Autodesk Fusion 360 part; units mm, degrees
sketch "Sketch1" plane through (0, 0, 0) normal (0, 0, 1) x (1, 0, 0)
  line L0 (0, 0) -> (100, 0)
  line L1 (100, 0) -> (100, 100)
  line L2 (100, 100) -> (0, 100)
  line L3 (0, 100) -> (0, 0)
  line L4 (0, 0) -> (15, 0)
  line L5 (15, 0) -> (15, 15)
  line L6 (100, 100) -> (85, 100)
  line L7 (85, 100) -> (85, 85)
  line L8 (15, 15) -> (85, 15)
  line L9 (85, 15) -> (85, 85)
  line L10 (85, 85) -> (15, 85)
  line L11 (15, 85) -> (15, 15)
  dimension "d1" = 100
  dimension "d2" = 100
  dimension "d3" = 15
  dimension "d4" = 15
  dimension "d5" = 15
  dimension "d6" = 15
extrude "Extrude1" add sketch "Sketch1" along normal blind 5 contours L0 L2 L3 L4 L5 L7 L10 L11 | L0 L1 L2 L5 L6 L7 L8 L9
chamfer "Chamfer1" distance 5 angle 45 1 edges at (50, 0, 5)
chamfer "Chamfer2" distance 5 angle 45 1 edges at (0, 52.5, 5)
chamfer "Chamfer3" distance 5 angle 45 1 edges at (52.5, 100, 5)
chamfer "Chamfer4" distance 5 angle 45 1 edges at (100, 50, 5)
extrude "Extrude2" cut 1 faces at (5, 61.6667, 0) along direction (0, 0, 1) blind 3
sketch "Sketch2" plane through (0, 0, 5) normal (0, 0, 1) x (-1, 0, 0)
  line L0 (-15, -15) -> (-15, -85)
  line L1 (-15, -85) -> (-85, -85)
  line L2 (-85, -85) -> (-85, -15)
  line L3 (-85, -15) -> (-15, -15)
  line L4 (-95, -5) -> (-95, -95)
  line L5 (-95, -95) -> (-5, -95)
  line L6 (-5, -95) -> (-5, -5)
  line L7 (-5, -5) -> (-95, -5)
  circle A0 centre (-10, -90) radius 2.5
  line L8 (-10, -90) -> (-20, -90)
  circle A1 centre (-20, -90) radius 2.5
  line L9 (-10, -90) -> (-10, -80)
  circle A2 centre (-10, -80) radius 2.5
  circle A3 centre (-90, -90) radius 2.5
  line L10 (-90, -90) -> (-90, -80)
  line L11 (-90, -90) -> (-80, -90)
  circle A4 centre (-90, -80) radius 2.5
  circle A5 centre (-80, -90) radius 2.5
  circle A6 centre (-90, -10) radius 2.5
  line L12 (-90, -10) -> (-90, -20)
  line L13 (-90, -10) -> (-80, -10)
  circle A7 centre (-80, -10) radius 2.5
  circle A8 centre (-90, -20) radius 2.5
  circle A9 centre (-10, -10) radius 2.5
  line L14 (-10, -10) -> (-20, -10)
  line L15 (-10, -10) -> (-10, -20)
  circle A10 centre (-20, -10) radius 2.5
  circle A11 centre (-10, -20) radius 2.5
  dimension "d15" = 5
  dimension "d16" = 10
  dimension "d17" = 5
  dimension "d18" = 10
  dimension "d19" = 5
  dimension "d20" = 5
  dimension "d21" = 10
  dimension "d22" = 10
  dimension "d23" = 5
  dimension "d24" = 5
  dimension "d25" = 5
  dimension "d26" = 10
  dimension "d27" = 10
  dimension "d28" = 5
  dimension "d29" = 5
  dimension "d30" = 5
  dimension "d31" = 10
  dimension "d32" = 10
  dimension "d33" = 5
  dimension "d34" = 5
extrude "Extrude3" cut sketch "Sketch2" against normal blind 5 contours A0 L8 L9 | A1 | A2 | A0 L8 L9 | A3 L10 L11 | A4 | A3 L10 L11 | A5 | A6 L12 L13 | A8 | A6 L12 L13 | A7 | A9 L14 L15 | A11 | A10 | A9 L14 L15
fillet "Fillet1" radius 5 1 edges at (15, 85, 4)
fillet "Fillet2" radius 5 1 edges at (85, 15, 4)
fillet "Fillet3" radius 5 1 edges at (15, 15, 4)
fillet "Fillet4" radius 5 1 edges at (85, 85, 4)
Build history of the part. All positions in model axes, mm. A direction names the side the tool comes from. Coordinates: 2 decimals unless noted, no trailing zeros. Order: outer loops, then holes, each group sorted by start corner. A loop starts at its lowest first (then second) coordinate and runs counter-clockwise, first axis right, second up. Notation, with made-up numbers: M 18.25,-39 L 50.25,-39 A34 cw 50.25,-1 Z; hole C 30,54.25 d3. An arc over 180 degrees is marked long. One line per question, with ' | ' between items. Start each with the question number.
1. Cut at A-A (x = 57). Write the cut outline in (y, z), plus the area to 3 significant figures.
2. Cut at C-C (x = 90). Write the cut outline in (y, z).
3. Mould opens along Y. For faces 1 (the face through (51, 4, 4)), 2 (the face through (49, 96, 4)), 3 (the face through (92.5, 79.9, 4)) say: +Y half, -Y half, draft (parallel to the pull), parting line (faces both ways), or undercut.
4. Tool access for faces 4 (the face through (4, 49, 4)), 5 (the face through (17, 84, 4)): list every direction of +Z, -Z, +X, -X, +Y, -Y with a clear straight run to the whole face (end or side of a thin tool).
5. Wall check: line 1 along X through (y, z) = (10, 4.9); line 2 along X through (y, z) = (20.5, 3.95); line 3 along X through (y, z) = (10, 3.65). Give the ranges that are in metal, low to high. Write a range as [from, to].
6. Flat gauge pins, fed straight in: P1, Ø3, axis at x = 90, y = 10, coming from the +Z side; P2, Ø0.6, axis at y = 40, z = 4, coming from the +X side; P3, Ø0.6, axis at y = 44, z = 3.5, coming from the -X side; P4, Ø0.6, axis at x = 45, z = 4, coming from the -Y side. Where does each tip first touch, or does it go through?
The answers:
1) outline: M 3,3 L 15,3 L 15,5 L 5,5 Z; M 85,3 L 97,3 L 95,5 L 85,5 Z | area: 44.0 mm2
2) outline: M 3,3 L 7.5,3 L 7.5,5 L 5,5 Z; M 12.5,3 L 17.5,3 L 17.5,5 L 12.5,5 Z; M 22.5,3 L 77.5,3 L 77.5,5 L 22.5,5 Z; M 82.5,3 L 87.5,3 L 87.5,5 L 82.5,5 Z; M 92.5,3 L 97,3 L 95,5 L 92.5,5 Z
3) face 1: -Y half | face 2: +Y half | face 3: undercut
4) face 4: +Z, -X, +Y, -Y | face 5: +Z, -Z
5) line 1: x = [4.9, 7.5], [12.5, 17.5], [22.5, 77.5], [82.5, 87.5], [92.5, 95.1] | line 2: x = [3.95, 7.55], [12.45, 15], [85, 87.55], [92.45, 96.05] | line 3: x = [3.65, 7.5], [12.5, 17.5], [22.5, 77.5], [82.5, 87.5], [92.5, 96.35]
6) P1: passes through | P2: stops at x = 96.3 | P3: stops at x = 3.2 | P4: stops at y = 3.7
